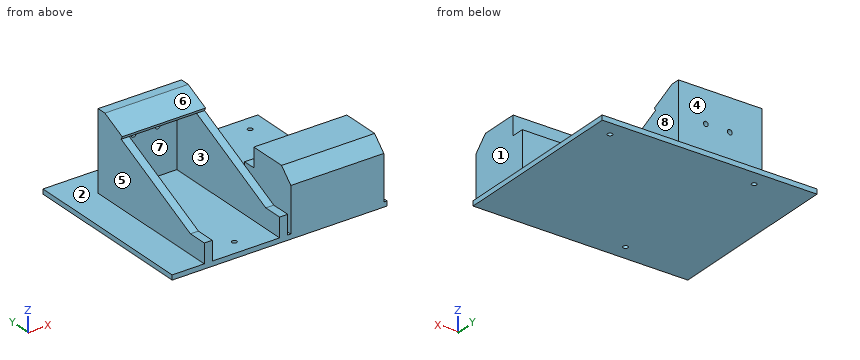
```python
from build123d import *

# Parameters (mm, degrees)
SKETCH1_W           = 72
SKETCH1_H           = 92
BOSS_EXTRUDE1_DEPTH = 3
SKETCH2_W           = 5
SKETCH2_H           = 92
BOSS_EXTRUDE2_DEPTH = 47
BOSS_EXTRUDE3_REACH = 52
SKETCH3_W           = 52
SKETCH3_H           = 20
CUT_EXTRUDE3_REACH  = 54
SKETCH8_W           = 52
SKETCH8_H           = 16.552945357
BOSS_EXTRUDE5_DEPTH = 2
SKETCH9_W           = 52
SKETCH9_H           = 5
SKETCH9_H_2         = 0.845770931
BOSS_EXTRUDE6_DEPTH = 1.812366
SKETCH10_W          = 42
SKETCH10_H          = 40
CUT_EXTRUDE4_DEPTH  = 17
CUT_EXTRUDE5_REACH  = 94
SKETCH12_R          = 1.5
SKETCH13_W          = 72
SKETCH13_H          = 3
BOSS_EXTRUDE7_DEPTH = 20
SKETCH15_W          = 3
SKETCH15_H          = 112
BOSS_EXTRUDE8_DEPTH = 62
SKETCH17_W          = 58
SKETCH17_H          = 40
BOSS_EXTRUDE9_DEPTH = 36
CHAMFER1_SIZE       = 8
SKETCH18_W          = 58
SKETCH18_H          = 8
CUT_EXTRUDE8_DEPTH  = 12
CUT_EXTRUDE9_REACH  = 5
SKETCH14_R          = 1.5


with BuildPart() as part:
    # Sketch1 → Boss-Extrude1 (new body)
    with BuildSketch(Plane.XY):
        Rectangle(SKETCH1_W, SKETCH1_H)
    extrude(amount=BOSS_EXTRUDE1_DEPTH)

    # Sketch2 → Boss-Extrude2 (add)
    with BuildSketch(Plane.XY.offset(3)):
        with Locations((33.5, 0)):
            Rectangle(SKETCH2_W, SKETCH2_H)
        with Locations((-13.5, 0)):
            Rectangle(SKETCH2_W, SKETCH2_H)
    extrude(amount=BOSS_EXTRUDE2_DEPTH)

    # Sketch3 → Boss-Extrude3 (add, up to next)
    with BuildSketch(Plane.XY.offset(50), mode=Mode.PRIVATE) as boss_extrude3_sk1:
        with Locations((10, 36)):
            Rectangle(SKETCH3_W, SKETCH3_H)
    boss_extrude3_tool1 = extrude(boss_extrude3_sk1.sketch, amount=-BOSS_EXTRUDE3_REACH, mode=Mode.PRIVATE) - part.part
    add(boss_extrude3_tool1.solids().sort_by_distance((10, 36, 50))[0])

    # Sketch7 → Cut-Extrude3 (cut, up to next)
    with BuildSketch(Plane.ZY.offset(16), mode=Mode.PRIVATE) as cut_extrude3_sk1:
        Polygon((50, 41), (15, -34), (15, -46), (50, -46), align=None)
    cut_extrude3_tool1 = extrude(cut_extrude3_sk1.sketch, amount=-CUT_EXTRUDE3_REACH, mode=Mode.PRIVATE) & part.part
    add(cut_extrude3_tool1.solids().sort_by_distance((-16, -16.515152, 36.919192))[0], mode=Mode.SUBTRACT)

    # Sketch8 → Boss-Extrude5 (add)
    with BuildSketch(Plane(origin=(0, -11.828467153, 25.346715328), x_dir=(1, 0, 0), z_dir=(0, -0.422885465, 0.90618314))):
        with Locations((10, 50.021309328)):
            Rectangle(SKETCH8_W, SKETCH8_H)
    extrude(amount=BOSS_EXTRUDE5_DEPTH)

    # Sketch9 → Boss-Extrude6 (add)
    with BuildSketch(Plane.XY.offset(50)):
        with Locations((10, 43.5)):
            Rectangle(SKETCH9_W, SKETCH9_H)
        with Locations((10, 40.577114534)):
            Rectangle(SKETCH9_W, SKETCH9_H_2)
    extrude(amount=BOSS_EXTRUDE6_DEPTH)

    # Sketch10 → Cut-Extrude4 (cut)
    with BuildSketch(Plane.XZ.offset(-26)):
        with Locations((10, 23)):
            Rectangle(SKETCH10_W, SKETCH10_H)
    extrude(amount=-CUT_EXTRUDE4_DEPTH, mode=Mode.SUBTRACT)

    # Sketch12 → Cut-Extrude5 (cut, up to next)
    with BuildSketch(Plane(origin=(0, 46, 0), x_dir=(1, 0, 0), z_dir=(0, 1, 0)), mode=Mode.PRIVATE) as cut_extrude5_sk1:
        with Locations((4, -31.81236628)):
            Circle(SKETCH12_R)
    cut_extrude5_tool1 = extrude(cut_extrude5_sk1.sketch, amount=-CUT_EXTRUDE5_REACH, mode=Mode.PRIVATE) & part.part
    add(cut_extrude5_tool1.solids().sort_by_distance((4, 46, 31.812366))[0], mode=Mode.SUBTRACT)
    # Sketch12 → Cut-Extrude5 (cut, up to next)
    with BuildSketch(Plane(origin=(0, 46, 0), x_dir=(1, 0, 0), z_dir=(0, 1, 0)), mode=Mode.PRIVATE) as cut_extrude5_sk2:
        with Locations((19, -31.81236628)):
            Circle(SKETCH12_R)
    cut_extrude5_tool2 = extrude(cut_extrude5_sk2.sketch, amount=-CUT_EXTRUDE5_REACH, mode=Mode.PRIVATE) & part.part
    add(cut_extrude5_tool2.solids().sort_by_distance((19, 46, 31.812366))[0], mode=Mode.SUBTRACT)

    # Sketch13 → Boss-Extrude7 (add)
    with BuildSketch(Plane(origin=(0, 46, 0), x_dir=(1, 0, 0), z_dir=(0, 1, 0))):
        with Locations((0, -1.5)):
            Rectangle(SKETCH13_W, SKETCH13_H)
    extrude(amount=BOSS_EXTRUDE7_DEPTH)

    # Sketch15 → Boss-Extrude8 (add)
    with BuildSketch(Plane(origin=(36, 0, 0), x_dir=(0, 0, -1), z_dir=(1, 0, 0))):
        with Locations((-1.5, 10)):
            Rectangle(SKETCH15_W, SKETCH15_H)
    extrude(amount=BOSS_EXTRUDE8_DEPTH)

    # Sketch17 → Boss-Extrude9 (add)
    with BuildSketch(Plane.XY.offset(3)):
        with Locations((67, -26)):
            Rectangle(SKETCH17_W, SKETCH17_H)
    extrude(amount=BOSS_EXTRUDE9_DEPTH)

    # Chamfer1
    chamfer1_edges = [part.edges().sort_by_distance(p)[0] for p in [
        (67, -46, 39),
    ]]
    chamfer(chamfer1_edges, length=CHAMFER1_SIZE)

    # Sketch18 → Cut-Extrude8 (cut)
    with BuildSketch(Plane.XY.offset(39)):
        with Locations((67, -10)):
            Rectangle(SKETCH18_W, SKETCH18_H)
    extrude(amount=-CUT_EXTRUDE8_DEPTH, mode=Mode.SUBTRACT)

    # Sketch14 → Cut-Extrude9 (cut, up to next)
    with BuildSketch(Plane.XY.offset(3), mode=Mode.PRIVATE) as cut_extrude9_sk1:
        with Locations((86, 56)):
            Circle(SKETCH14_R)
    cut_extrude9_tool1 = extrude(cut_extrude9_sk1.sketch, amount=-CUT_EXTRUDE9_REACH, mode=Mode.PRIVATE) & part.part
    add(cut_extrude9_tool1.solids().sort_by_distance((86, 56, 3))[0], mode=Mode.SUBTRACT)
    # Sketch14 → Cut-Extrude9 (cut, up to next)
    with BuildSketch(Plane.XY.offset(3), mode=Mode.PRIVATE) as cut_extrude9_sk2:
        with Locations((10, -36)):
            Circle(SKETCH14_R)
    cut_extrude9_tool2 = extrude(cut_extrude9_sk2.sketch, amount=-CUT_EXTRUDE9_REACH, mode=Mode.PRIVATE) & part.part
    add(cut_extrude9_tool2.solids().sort_by_distance((10, -36, 3))[0], mode=Mode.SUBTRACT)
    # Sketch14 → Cut-Extrude9 (cut, up to next)
    with BuildSketch(Plane.XY.offset(3), mode=Mode.PRIVATE) as cut_extrude9_sk3:
        with Locations((-4, 56)):
            Circle(SKETCH14_R)
    cut_extrude9_tool3 = extrude(cut_extrude9_sk3.sketch, amount=-CUT_EXTRUDE9_REACH, mode=Mode.PRIVATE) & part.part
    add(cut_extrude9_tool3.solids().sort_by_distance((-4, 56, 3))[0], mode=Mode.SUBTRACT)


solid = part.part
```
The listing builds one solid part. Answer for the finished solid, in the listing's coordinates (mm). Face numbers are marked on the shaded views. A direction names the side the tool comes from. Round coordinates to 2 decimals unless told otherwise and drop trailing zeros. Loops run counter-clockwise (first coordinate to the right, second up) from the corner with the lowest first, then second, coordinate; pieces in that order, holes last.
Q1. Find the intervals of material crossed by line 1 (Y direction, x = 10, z = 1.7); line 2 (Z direction, x = 19, y = 44); line 3 (X direction, y = 15, z = 34.5), in increasing order.
Q2. Given pin 1 Ø1.5 at (x, z) = (26, 37.5) entering from -Y; pin 2 Ø20 at (y, z) = (-4, 22.5) entering from -X; pin 3 Ø24.5 at (y, z) = (-22, 26) entering from +X, each flat-ended and moving along its own axis, determine where each tip first touches the part or whether it passes through.
Q3. Section C-C, the plane z = 22 is taken. Determine the outline of the cut face in (x, y), then the cut area to 3 significant figures.
Q4. Section D-D, the plane y = 56 is taken. Determine the outline of the cut face in (x, z).
Q5. For a pull along Z with two mould halves and no side action, classify the marked faces 6, 7 and 8 as released by +Z, released by -Z, zero draft, split by the parting line, or undercut.
Q6. Section A-A, the plane x = 19 is taken. Determine the outline of the cut face in (y, z), then the cut area to 3 significant figures.
Q7. Which of the six approach directions +Z, -Z, +X, -X, +Y, -Y give full straight-line access (tool end or side, diameter ignored) to the marked faces 1, 2, 3, 4 and 5?
Q8. Section B-B, the plane y = -36 is taken. Determine the outline of the cut face in (x, z), then the cut area to 3 significant figures.
Completed:
1. line 1: y = -46 to -37.5, -34.5 to 66
1. line 2: z = 0 to 30.31, 33.31 to 51.81
1. line 3: x = -16 to -11, 31 to 36
2. pin 1: stops at y = 43
2. pin 2: stops at x = -16
2. pin 3: stops at x = 96
3. outline: (-16, -19) - (-11, -19) - (-11, 43) - (31, 43) - (31, -19) - (36, -19) - (36, 46) - (-16, 46) - close; (38, -46) - (96, -46) - (96, -6) - (38, -6) - close
3. area: 3,100 mm2
4. outline: (-36, 0) - (-5.5, 0) - (-5.5, 3) - (-36, 3) - close; (-2.5, 0) - (84.5, 0) - (84.5, 3) - (-2.5, 3) - close; (87.5, 0) - (98, 0) - (98, 3) - (87.5, 3) - close
5. face 6: released by +Z
5. face 7: undercut
5. face 8: zero draft
6. outline: (-46, 0) - (66, 0) - (66, 3) - (46, 3) - (46, 30.31) - (43, 30.31) - (43, 3) - (-46, 3) - close; (25.15, 44.81) - (26, 43) - (43, 43) - (43, 33.31) - (46, 33.31) - (46, 51.81) - (40.15, 51.81) - close
6. area: 577 mm2
7. face 1: +Z, +X, +Y, -Y
7. face 2: +Z, +Y
7. face 3: -Y
7. face 4: +Z, +X, -X, +Y
7. face 5: +Z, -X, +Y, -Y
8. outline: (-36, 0) - (8.5, 0) - (8.5, 3) - (-11, 3) - (-11, 15) - (-16, 15) - (-16, 3) - (-36, 3) - close; (11.5, 0) - (98, 0) - (98, 3) - (96, 3) - (96, 39) - (38, 39) - (38, 3) - (36, 3) - (36, 15) - (31, 15) - (31, 3) - (11.5, 3) - close
8. area: 2,600 mm2
